The figure shows three views and two pictorial views of one solid part (mm, origin at its lowest corner). Answer the questions. Round coordinates to 2 decimals unless told otherwise and drop trailing zeros. Loops run counter-clockwise (first coordinate to the right, second up) from the corner with the lowest first, then second, coordinate; pieces in that order, holes last. Notation, with made-up numbers: (53, 35.25) -> (80, 35.25) arc R6 ccw to (80, 39.25) -> close; hole circle Ø5 at (-9.5, -4.5). An arc over 180 degrees is marked (long way). Write each question's results on one line, items separated by ' | '. Start each with the question number.
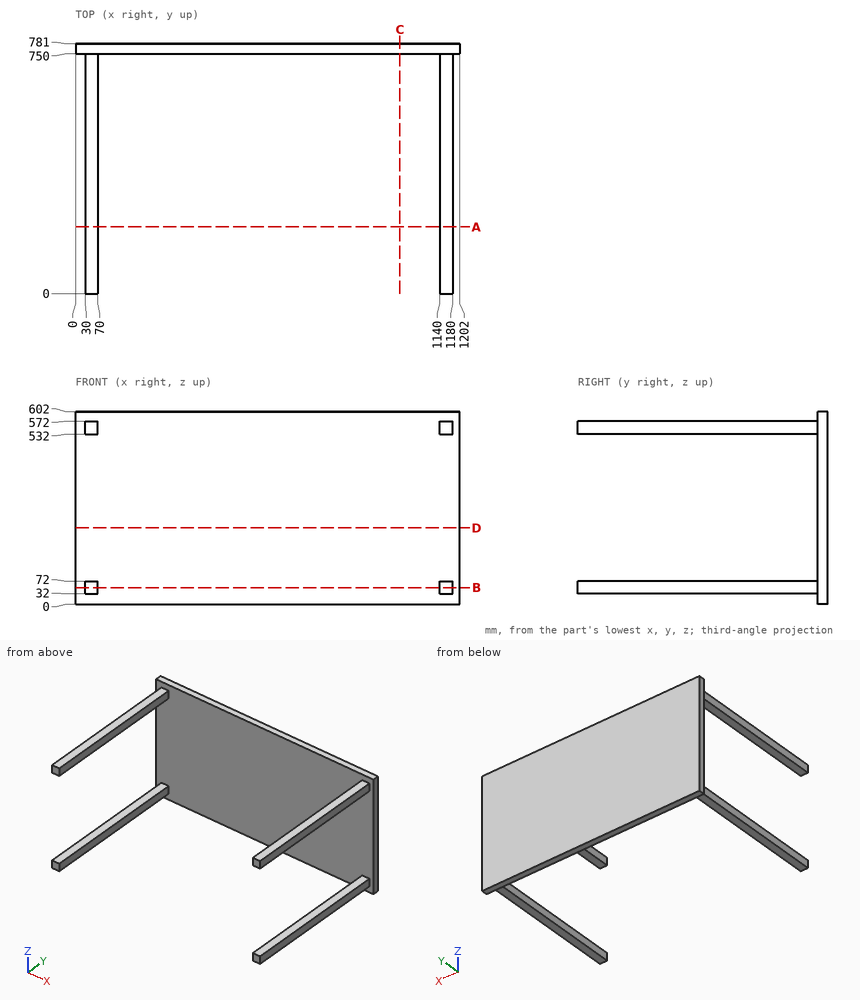
Item 1: The part is cut by section C-C, the plane x = 1014.5. Give the vertices of the cut face in (y, z), plus the area to 3 significant figures.
Item 2: Straight lines are drawn through the part: L1, parallel to X at y = 466.5, z = 566.5; L2, parallel to Y at x = 476.5, z = 403.5. For each, find the intervals that lie inside material, in ascending order. Write a range as [from, to].
Item 3: The part is cut by section A-A, the plane y = 209. Give the vertices of the cut face in (x, z).
Item 4: Each of these flat-tipped pins is pushed along its axis until it touches: pin 1 Ø1 at (x, z) = (869.5, 466.5) entering from -Y; pin 2 Ø10 at (y, z) = (576.5, 68.5) entering from +X; pin 3 Ø12 at (y, z) = (416, 556) entering from -X. Where does it stop, or does it pass through?
Item 5: The part is cut by section D-D, the plane z = 239. Give the vertices of the cut face in (x, y).
Item 6: The part is cut by section B-B, the plane z = 51.5. Give the vertices of the cut face in (x, y).
Report:
1) outline: (750, 0) -> (781, 0) -> (781, 602) -> (750, 602) -> close | area: 18,700 mm2
2) L1: x = [30, 70], [1140, 1180] | L2: y = [750, 781]
3) outline: (30, 32) -> (70, 32) -> (70, 72) -> (30, 72) -> close; (30, 532) -> (70, 532) -> (70, 572) -> (30, 572) -> close; (1140, 32) -> (1180, 32) -> (1180, 72) -> (1140, 72) -> close; (1140, 532) -> (1180, 532) -> (1180, 572) -> (1140, 572) -> close
4) pin 1: stops at y = 750 | pin 2: stops at x = 1180 | pin 3: stops at x = 30
5) outline: (0, 750) -> (1202, 750) -> (1202, 781) -> (0, 781) -> close
6) outline: (0, 750) -> (30, 750) -> (30, 0) -> (70, 0) -> (70, 750) -> (1140, 750) -> (1140, 0) -> (1180, 0) -> (1180, 750) -> (1202, 750) -> (1202, 781) -> (0, 781) -> close
